Can you work these out from the model? Positions are in its coordinate system, mm. A direction names the side the tool comes from. Round coordinates to 2 decimals unless told otherwise and drop trailing zeros. Loops run counter-clockwise (first coordinate to the right, second up) from the corner with the lowest first, then second, coordinate; pieces in that order, holes last.
from build123d import *


with BuildPart() as f1:
    # F0 (on Front) → F1 (revolve)
    with BuildSketch(Plane.XZ):
        with BuildLine():
            Line((7.5, -15), (7.5, -4))
            ThreePointArc((7.5, -4), (6.328427, -1.171573), (3.5, 0))
            Line((3.5, 0), (0, 0))
            Line((0, 0), (0, -100))
            Line((0, -100), (9.5, -100))
            Line((9.5, -100), (9.5, -65))
            Line((9.5, -65), (7.5, -60))
            Line((7.5, -60), (7.5, -53.465673))
            ThreePointArc((7.5, -53.465673), (6.474874, -50.990799), (4, -49.965673))
            Line((4, -49.965673), (4, -34))
            Line((4, -34), (7.5, -15))
        make_face()
    revolve(axis=Axis((0, 0, -50), (0, 0, 1)))


solid = f1.part
(1) Will these pins go through, and if not, where does the flat tip stop? P1, Ø8, axis at x = -3.5, z = -45, coming from the -Y side; P2, Ø5, axis at x = -3, y = 6, coming from the +Z side; P3, Ø2, axis at x = 7.5, z = -80, coming from the -Y side.
Worked answers:
P1: stops at y = -4
P2: stops at z = -0.06
P3: stops at y = -6.93
(2) If I drill on line 1 (X direction, y = -3.25, z = -86.5); line 2 (Z direction, x = -7.75, y = 4); line 3 (X direction, y = 1.5, z = -34.5), over which ranges is the centre line in solid material (lowest first)?
Worked answers:
line 1: x = -8.93 to 8.93
line 2: z = -100 to -63.05
line 3: x = -3.71 to 3.71
(3) For faces 1 (the conical face through (-5.77, 0.25, -24.37)), 2 (the cylindrical face through (-7.493, 0.33, -56.687)), 3 (the flat face through (0, 0, -100)), which set-ups out of +Z, -Z, +X, -X, +Y, -Y let a thin tool reach every point of the face, with its end or its side?
Worked answers:
face 1: none
face 2: +Z
face 3: -Z, +X, -X, +Y, -Y
(4) If we section it at A-A, the plane z = -36.5: List the corners of the cut face in (x, y) for me, then the cut area to 3 significant figures.
Worked answers:
outline: circle Ø8 at (0, 0)
area: 50.3 mm2
(5) If we section it at B-B, the plane z = -10: List the corners of the cut face in (x, y) for me.
Worked answers:
outline: circle Ø15 at (0, 0)
